The figure shows three views and two pictorial views of one solid part (mm, origin at its lowest corner). Answer the questions. A direction names the side the tool comes from. Round coordinates to 2 decimals unless told otherwise and drop trailing zeros. Write each loop counter-clockwise with the first axis right and the second up, starting at its lowest first coordinate (ties: lowest second). Pieces come first, ordered by that corner, then holes. Notation, with made-up numbers: M -23.75,74.5 L -8.75,74.5 A23 ccw -8.75,87.5 Z; hole C 3.5,-29.75 d3. An arc over 180 degrees is marked long. Answer in a Markdown table with one row per item.
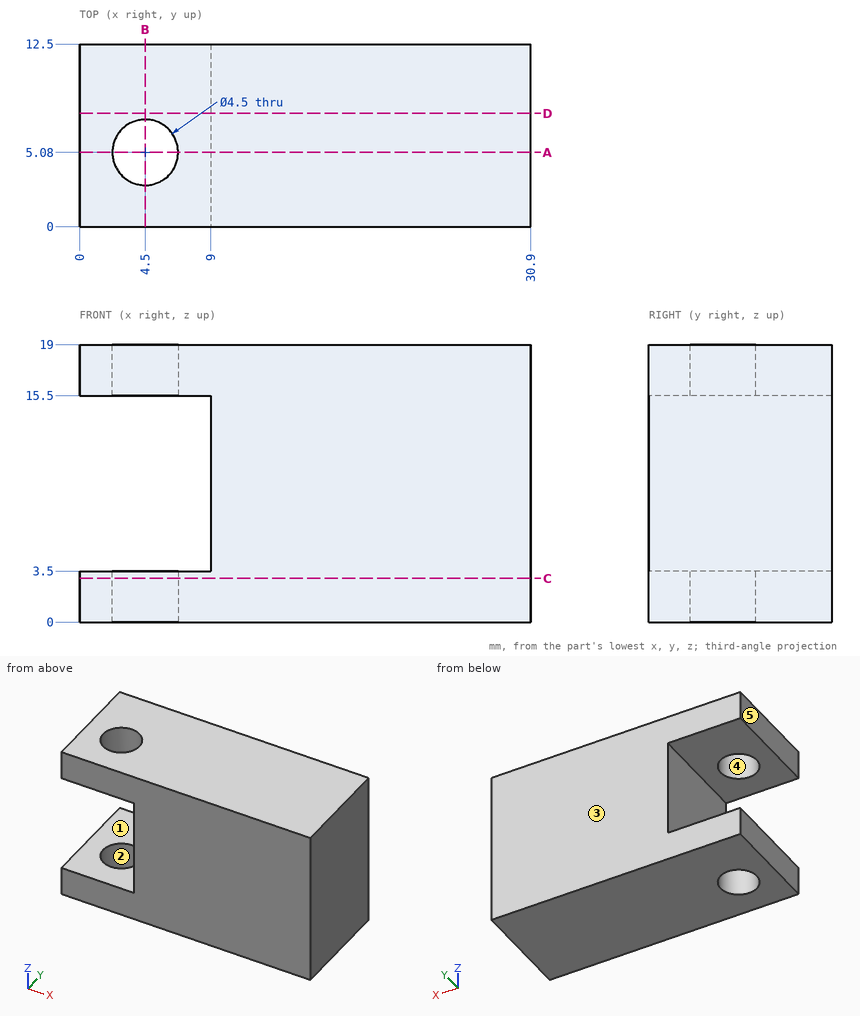
1. Determine the mould class of the marked faces 3, 4 and 5 for opening direction Y: released by +Y, released by -Y, zero draft, split by the parting line, or undercut.
Calculated:
| item | result |
|---|---|
| face 3 | released by +Y |
| face 4 | undercut |
| face 5 | zero draft |
2. The part is cut by section B-B (x = 4.5). Determine the outline of the cut face in (y, z), plus the area to 3 significant figures.
Calculated:
| item | result |
|---|---|
| outline | M 0,0 L 2.83,0 L 2.83,3.5 L 0,3.5 Z; M 0,15.5 L 2.83,15.5 L 2.83,19 L 0,19 Z; M 7.33,0 L 12.5,0 L 12.5,3.5 L 7.33,3.5 Z; M 7.33,15.5 L 12.5,15.5 L 12.5,19 L 7.33,19 Z |
| area | 56.0 mm² |
3. The part is cut by section A-A (y = 5.08). Determine the outline of the cut face in (x, z), plus the area to 3 significant figures.
Calculated:
| item | result |
|---|---|
| outline | M 0,0 L 2.25,0 L 2.25,3.5 L 0,3.5 Z; M 0,15.5 L 2.25,15.5 L 2.25,19 L 0,19 Z; M 6.75,0 L 30.9,0 L 30.9,19 L 6.75,19 L 6.75,15.5 L 9,15.5 L 9,3.5 L 6.75,3.5 Z |
| area | 448 mm² |
4. The part is cut by section C-C (z = 3). Determine the outline of the cut face in (x, y).
Calculated:
| item | result |
|---|---|
| outline | M 0,0 L 30.9,0 L 30.9,12.5 L 0,12.5 Z; hole C 4.5,5.08 d4.5 |
5. The part is cut by section D-D (y = 7.75). Determine the outline of the cut face in (x, z), plus the area to 3 significant figures.
Calculated:
| item | result |
|---|---|
| outline | M 0,0 L 30.9,0 L 30.9,19 L 0,19 L 0,15.5 L 9,15.5 L 9,3.5 L 0,3.5 Z |
| area | 479 mm² |
6. A tool of negligible diameter and unlimited length cuts with its end or side. For the marked faces 1 and 2, from which of +Z, -Z, +X, -X, +Y, -Y can it reach the whole face along a straight path? Write none if from no direction.
Calculated:
| item | result |
|---|---|
| face 1 | -X, +Y, -Y |
| face 2 | +Z, -Z |
7. Given pin 1 (6 mm diameter, centred on y = 4.5, z = 10.5, fed in from -X), flat-ended and moving along its own axis, determine where the tip first touches the part or whether it passes through.
Calculated:
| item | result |
|---|---|
| pin 1 | stops at x = 9 |
8. Consider line 1 along Y through (x, z) = (4.5, 16.7); line 2 along X through (y, z) = (9.25, 12.5). Determine where each line is inside the solid, lowest interval first. Write a range as from..to.
Calculated:
| item | result |
|---|---|
| line 1 | y = 0..2.83, 7.33..12.5 |
| line 2 | x = 9..30.9 |
